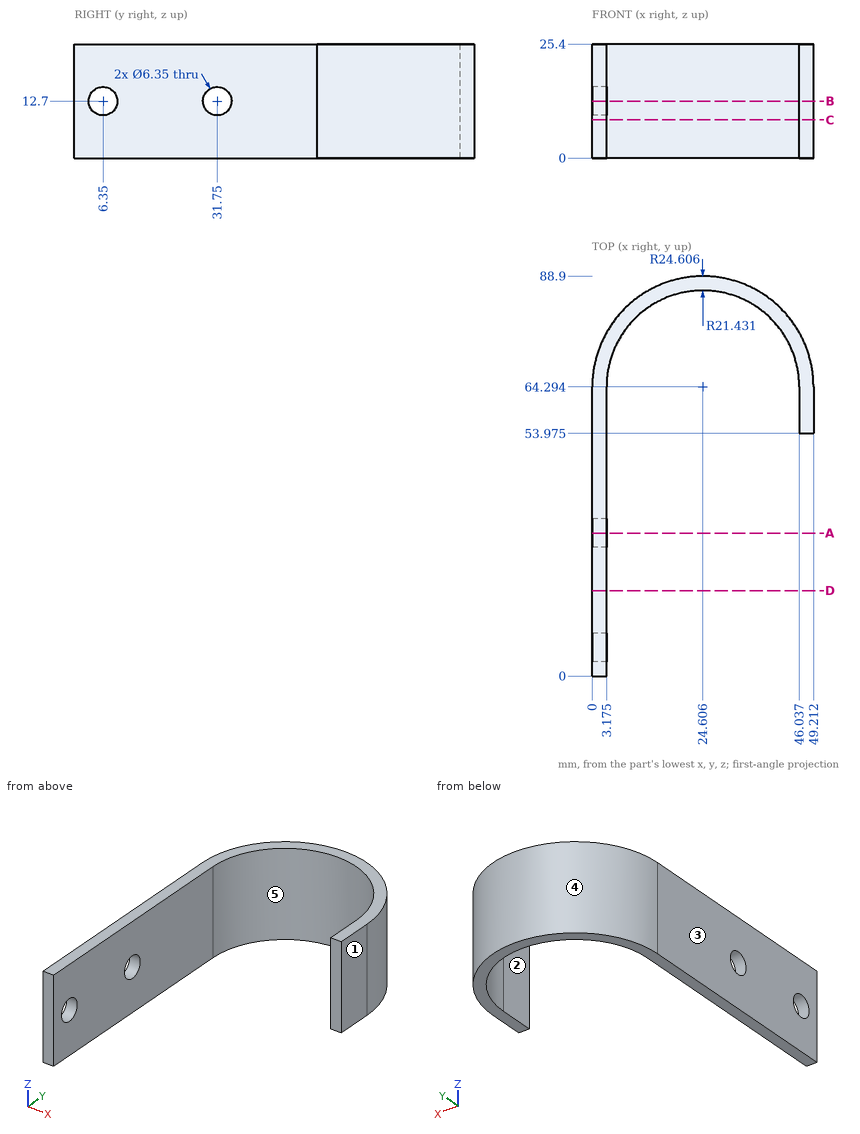
Verification items for this drawing (mm, ordinates from the low corner). A direction names the side the tool comes from. Coordinates: 2 decimals unless noted, no trailing zeros. Write each loop counter-clockwise with the first axis right and the second up, starting at its lowest first coordinate (ties: lowest second). Pieces come first, ordered by that corner, then holes. Notation, with made-up numbers: (-5.5, 83.5) -> (0.5, 83.5) arc R26 cw to (0.5, 100.5) -> close; hole circle Ø6 at (7, 52.25). An arc over 180 degrees is marked (long way). One line per item, written item: value. Start each with the question number.
Q1. Cross-section at D-D on y = 19. Enter the section's corners in (x, z) (1 decimal).
Q2. Mould release check, pull along Y, two halves, no side actions. Record for the marked faces 3, 4 and 5: pulls with the +Y half, pulls with the -Y half, needs draft (parallel to the pull), parting line crosses it, or undercut.
Q3. Cross-section at B-B on z = 12.7. Enter the section's corners in (x, y) (1 decimal), and give its area (3 significant figures).
Q4. Cross-section at C-C on z = 8.5. Enter the section's corners in (x, y) (1 decimal).
Q5. Thickness scan on L1, parallel to Z at x = 0.6, y = 31.75 (1 decimal); L2, parallel to X at y = 26.5, z = 12.25 (1 decimal); L3, parallel to X at y = 65, z = 19.75 (1 decimal). Record the ranges inside material, lowest first. Write a range as from..to.
Q6. Go/stop test with flat-tipped pins: P1, Ø1.5, axis at y = 43, z = 6.5, coming from the +X side (1 decimal); P2, Ø2, axis at x = 28.5, z = 21.5, coming from the -Y side; P3, Ø2, axis at x = 8.5, z = 20.5, coming from the +Y side. Record where each tip stops, or that it passes through.
Q7. Cross-section at A-A on y = 31.75. Enter the section's corners in (x, z) (1 decimal).
Q8. Access from +Z, -Z, +X, -X, +Y, -Y to the whole of each face (thin tool, end or side, straight path). Record for the marked faces 1 and 2.
Checked values:
1. outline: (0, 0) -> (3.2, 0) -> (3.2, 25.4) -> (0, 25.4) -> close
2. face 3: needs draft
2. face 4: pulls with the +Y half
2. face 5: pulls with the -Y half
3. outline: (0, 0) -> (3.2, 0) -> (3.2, 3.2) -> (0, 3.2) -> close; (0, 9.5) -> (3.2, 9.5) -> (3.2, 28.6) -> (0, 28.6) -> close; (0, 34.9) -> (3.2, 34.9) -> (3.2, 64.3) arc R21.4 cw to (46, 64.3) -> (46, 54) -> (49.2, 54) -> (49.2, 64.3) arc R24.6 ccw to (0, 64.3) -> close
3. area: 426 mm²
4. outline: (0, 0) -> (3.2, 0) -> (3.2, 64.3) arc R21.4 cw to (46, 64.3) -> (46, 54) -> (49.2, 54) -> (49.2, 64.3) arc R24.6 ccw to (0, 64.3) -> close
5. L1: z = 0..9.5, 15.9..25.4
5. L2: x = 0..3.2
5. L3: x = 0..3.2, 46..49.2
6. P1: stops at x = 3.2
6. P2: stops at y = 85.16
6. P3: stops at y = 83.72
7. outline: (0, 0) -> (3.2, 0) -> (3.2, 9.5) -> (0, 9.5) -> close; (0, 15.9) -> (3.2, 15.9) -> (3.2, 25.4) -> (0, 25.4) -> close
8. face 1: +Z, -Z, +X, +Y, -Y
8. face 2: +Z, -Z, -Y
